The model under review builds one solid part; all positions refer to its coordinate system, in mm. A direction names the side the tool comes from. Coordinates: 2 decimals unless noted, no trailing zeros. Write each loop counter-clockwise with the first axis right and the second up, starting at its lowest first coordinate (ties: lowest second). Pieces come first, ordered by that corner, then holes. Notation, with made-up numbers: (36, 81) - (44, 81) arc R23 cw to (44, 114) - close; hole circle Ø7 at (48.5, -29.5). An arc over 180 degrees is marked (long way). Return JSON: item names as keys, results as strings. Group by question number.
(1) We need section A-A on z = 0. State the section outline as (x, y) points.
(2) For pin 1 Ø1.9 at (x, y) = (100, 14) entering from -Z; pin 2 Ø6 at (x, y) = (122.5, 13) entering from +Z; pin 3 Ø8 at (x, y) = (184, -10.5) entering from -Z, all flat-tipped, find the tip position at first contact; note any pin that passes through.
(3) Tool access review of faces 4 (the face through (297.121, 6.703, 16.166)), 5 (the face through (200, -17, -3)): name each direction out of +Z, -Z, +X, -X, +Y, -Y from which nothing blocks a thin tool from reaching the whole face with its end or side.
(4) We need section B-B on x = 317.5. State the section outline as (y, z) points.
(5) Draft analysis for pull direction X (two halves, no side actions). For faces 1 (the face through (400, 0, 0)), 2 (the face through (71, 12.5, 0)), 3 (the face through (300.246, 1.652, -0.245)), state which applies: released by +X, released by -X, zero draft, split by the parting line, or undercut.
(6) We need section C-C on x = 230. State the section outline as (y, z) points.
(7) To check wall thickness, follow L1, parallel to X at y = 0, z = -4; L2, parallel to X at y = -3, z = -1; L3, parallel to Y at x = 295, z = 1. State the ranges of each line that lie inside material, in increasing order. Write a range as from..to.
(8) We need section D-D on x = 166.5. State the section outline as (y, z) points, then the cut area to 3 significant figures.
```python
from build123d import *

# Parameters (mm, degrees)
CHAMFER1_SIZE           = 3
CUT_EXTRUDE1_START      = 17
CUT_EXTRUDE1_DEPTH      = 4.5
CUT_EXTRUDE2_DEPTH      = 401.764893672
CUT_EXTRUDE2_DEPTH_BACK = 401.764893672
SKETCH3_R               = 5.5
CUT_EXTRUDE3_DEPTH      = 401.764893681
CUT_EXTRUDE3_DEPTH_BACK = 401.764893681
SKETCH4_R               = 5.5


with BuildPart() as part:
    # Sketch1 → Revolve1 (revolve)
    with BuildSketch(Plane.XY, mode=Mode.PRIVATE) as revolve1_sk:
        Polygon((0, 0), (400, 0), (400, 17.5), (200, 17.5), (200, 17), (0, 17), align=None)
    revolve(revolve1_sk.sketch.rotate(Axis((0, 0, 0), (1, 0, 0)), 90), axis=Axis((0, 0, 0), (1, 0, 0)))

    # Chamfer1
    chamfer1_edges = [part.edges().sort_by_distance(p)[0] for p in [
        (0, 0, -17),
        (400, 0, -17.5),
    ]]
    chamfer(chamfer1_edges, length=CHAMFER1_SIZE)

    # Sketch2 → Cut-Extrude1 (cut)
    with BuildSketch(Plane(origin=(0, 0, 0), x_dir=(1, 0, 0), z_dir=(0, 1, 0)).offset(CUT_EXTRUDE1_START)):
        with BuildLine():
            Line((0, 5), (135, 5))
            ThreePointArc((135, 5), (140, 0), (135, -5))
            Line((135, -5), (0, -5))
            Line((0, -5), (0, 5))
        make_face()
    extrude(amount=-CUT_EXTRUDE1_DEPTH, mode=Mode.SUBTRACT)

    # Sketch3 → Cut-Extrude2 (cut, two sides: drawn at the far end of the back side and taken through both)
    with BuildSketch(Plane(origin=(0, 0, 0), x_dir=(1, 0, 0), z_dir=(0, 1, 0)).offset(-CUT_EXTRUDE2_DEPTH_BACK)):
        with Locations(Location((230, 0, 0), (0, 0, 270))):
            Circle(SKETCH3_R)
    extrude(amount=CUT_EXTRUDE2_DEPTH + CUT_EXTRUDE2_DEPTH_BACK, mode=Mode.SUBTRACT)

    # Sketch4 → Cut-Extrude3 (cut, two sides: drawn at the far end of the back side and taken through both)
    with BuildSketch(Plane.XY.offset(-CUT_EXTRUDE3_DEPTH_BACK)):
        with Locations((295, 0)):
            Circle(SKETCH4_R)
    extrude(amount=CUT_EXTRUDE3_DEPTH + CUT_EXTRUDE3_DEPTH_BACK, mode=Mode.SUBTRACT)


solid = part.part
```
Ans:
{
 "1": {"outline": "(0, -14) - (3, -17) - (200, -17) - (200, -17.5) - (224.5, -17.5) - (224.5, 17.5) - (200, 17.5) - (200, 17) - (140, 17) - (140, 12.5) - (0, 12.5) - close; (235.5, -17.5) - (397, -17.5) - (400, -14.5) - (400, 14.5) - (397, 17.5) - (235.5, 17.5) - close; hole circle Ø11 at (295, 0)"},
 "2": {"pin 1": "z = -10.89", "pin 2": "z = 13.75", "pin 3": "z = -15.71"},
 "3": {"face 4": "+X, -X", "face 5": "-X"},
 "4": {"outline": "circle Ø35 at (0, 0)"},
 "5": {"face 1": "released by +X", "face 2": "zero draft", "face 3": "undercut"},
 "6": {"outline": "(-16.61, -5.5) arc R17.5 ccw to (16.61, -5.5) - close; (-16.61, 5.5) - (16.61, 5.5) arc R17.5 ccw to start"},
 "7": {"L1": "0..226.23, 233.77..289.5, 300.5..400", "L2": "0..224.59, 235.41..290.39, 299.61..400", "L3": "-17.47..-5.5, 5.5..17.47"},
 "8": {"outline": "circle Ø34 at (0, 0)", "area": "908 mm²"}
}
